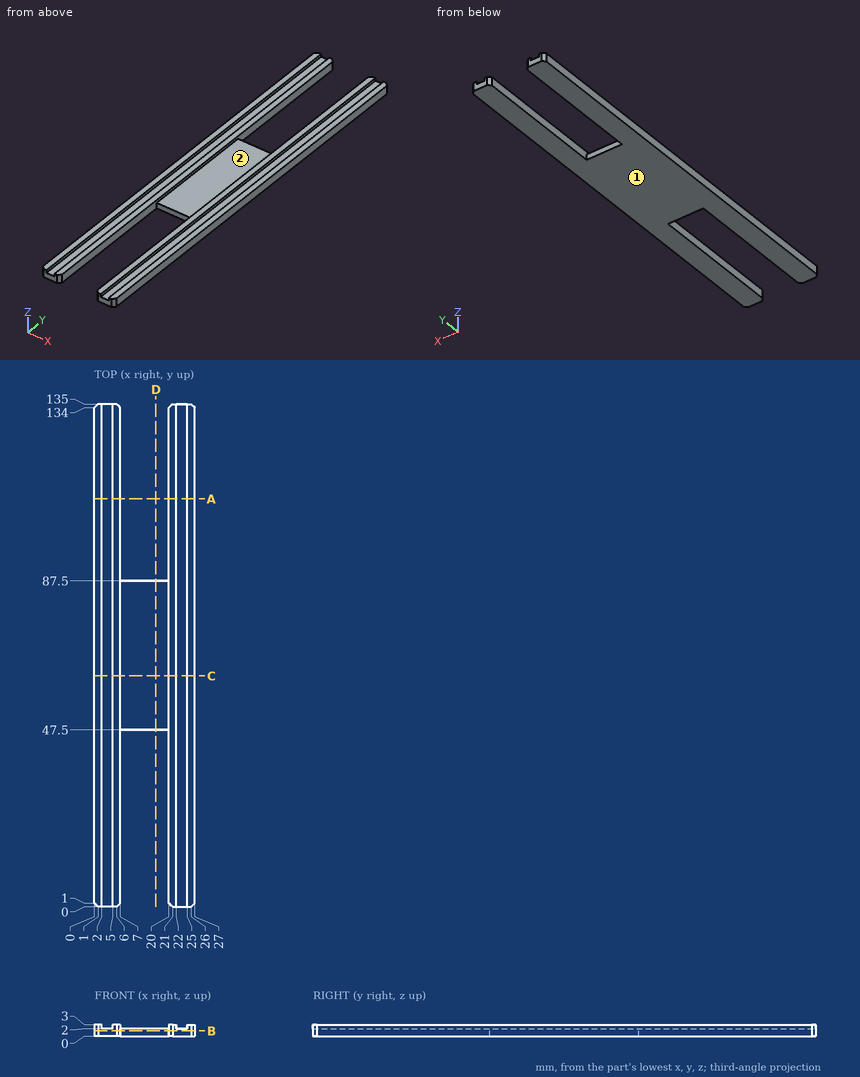
Verification items for this drawing (mm, ordinates from the low corner). Coordinates: 2 decimals unless noted, no trailing zeros. Write each loop counter-clockwise with the first axis right and the second up, starting at its lowest first coordinate (ties: lowest second). Pieces come first, ordered by that corner, then holes. Notation, with made-up numbers: M -38.75,57.5 L -1.75,57.5 A22 ccw -1.75,69.5 Z; hole C 63,16.25 d3. An arc over 180 degrees is marked long. Use one line per item in the form item = value. Start each with the question number.
1) Release check for a two-part mould opening along X. For the marked faces 1 and 2 record: pulls with the +X half, pulls with the -X half, needs draft (parallel to the pull), parting line crosses it, or undercut.
2) Go/stop test with a flat-tipped pin: pin 1 Ø1 at (x, z) = (13, 1.5) entering from -Y. Record where the tip stops, or that it passes through.
3) Thickness scan on probe 1 along X at (y, z) = (124.5, 2.3); probe 2 along X at (y, z) = (14, 1.7); probe 3 along Y at (x, z) = (17.75, 0.35). Record the ranges inside material, lowest first. Write a range as from..to.
4) Section check C-C on y = 62. Enter the section's corners in (x, z).
5) Section check B-B on z = 1.35. Enter the section's corners in (x, y), and give its area (3 significant figures).
6) Section check A-A on y = 109.5. Enter the section's corners in (x, z), and give its area (3 significant figures).
7) Section check D-D on x = 16.5. Enter the section's corners in (y, z), and give its area (3 significant figures).
Responses:
q1.face_1 = needs draft
q1.face_2 = undercut
q2.pin_1 = 47.5
q3.probe_1 = 0..2, 5..7, 20..22, 25..27
q3.probe_2 = 0..7, 20..27
q3.probe_3 = 47.5..87.5
q4.outline = M 0,0 L 27,0 L 27,3 L 25,3 L 25,2 L 22,2 L 22,3 L 20,3 L 20,2 L 7,2 L 7,3 L 5,3 L 5,2 L 2,2 L 2,3 L 0,3 Z
q5.outline = M 0,1 L 1,0 L 6,0 L 7,1 L 7,47.5 L 20,47.5 L 20,1 L 21,0 L 26,0 L 27,1 L 27,134 L 26,135 L 21,135 L 20,134 L 20,87.5 L 7,87.5 L 7,134 L 6,135 L 1,135 L 0,134 Z
q5.area = 2,410 mm2
q6.outline = M 0,0 L 7,0 L 7,3 L 5,3 L 5,2 L 2,2 L 2,3 L 0,3 Z; M 20,0 L 27,0 L 27,3 L 25,3 L 25,2 L 22,2 L 22,3 L 20,3 Z
q6.area = 36.0 mm2
q7.outline = M 47.5,0 L 87.5,0 L 87.5,2 L 47.5,2 Z
q7.area = 80.0 mm2
